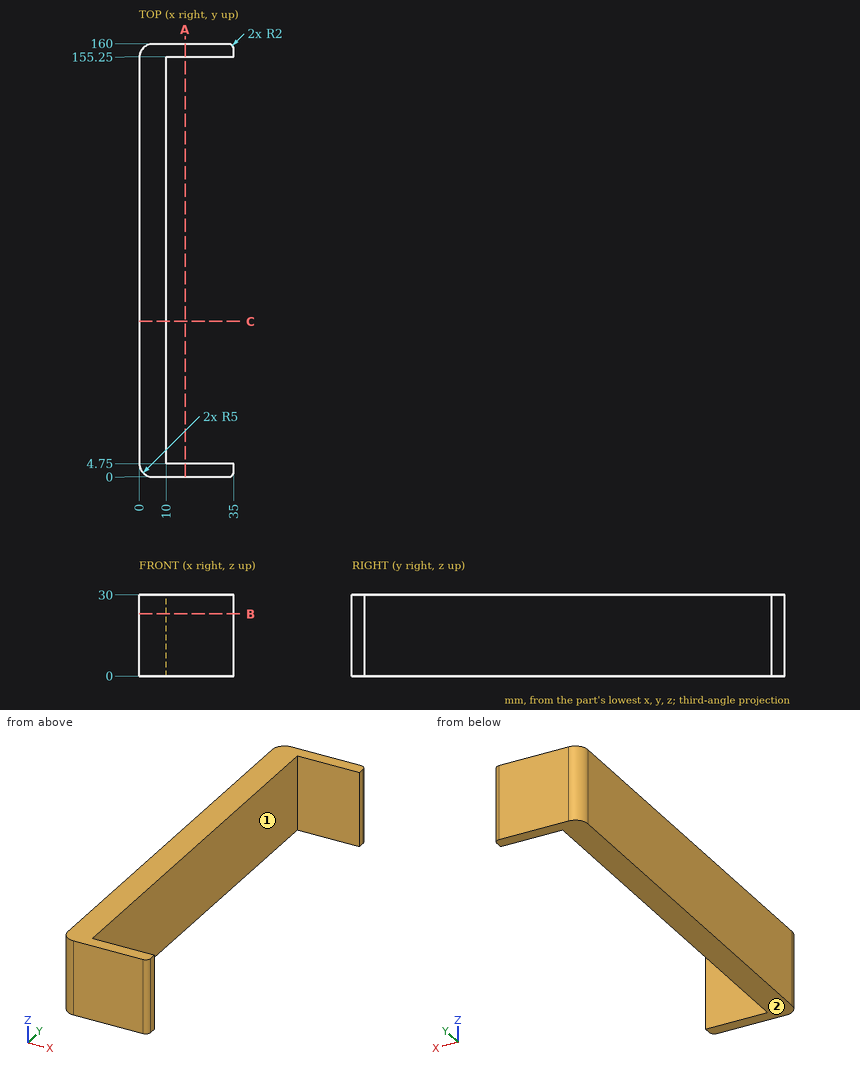
Verification items for this drawing (mm, ordinates from the low corner). A direction names the side the tool comes from. Give positions to 0.01 mm unless a question says otherwise; leave off trailing zeros. Write each loop counter-clockwise with the first axis right and the second up, starting at its lowest first coordinate (ties: lowest second). Pieces come first, ordered by that corner, then holes. Notation, with made-up numbers: (75, 27) -> (102, 27) arc R19 cw to (102, 50) -> close; hole circle Ø7 at (63, -18). An arc over 180 degrees is marked (long way). Use one line per item in the form item = value.
Item 1: Sectioned sample at B-B on z = 23. Enter the section's corners in (x, y), plus the area to 4 significant figures.
Results list:
outline = (0, 5) arc R5 ccw to (5, 0) -> (33, 0) arc R2 ccw to (35, 2) -> (35, 4.75) -> (10, 4.75) -> (10, 155.25) -> (35, 155.25) -> (35, 158) arc R2 ccw to (33, 160) -> (5, 160) arc R5 ccw to (0, 155) -> close
area = 1,825 mm2
Item 2: Sectioned sample at A-A on x = 17. Enter the section's corners in (y, z).
Results list:
outline = (0, 0) -> (4.75, 0) -> (4.75, 30) -> (0, 30) -> close; (155.25, 0) -> (160, 0) -> (160, 30) -> (155.25, 30) -> close
Item 3: Depth check by flat-ended pin: pin 1 Ø15 at (y, z) = (59, 18.5) entering from +X. Enter the tip coordinate at first touch or a pass-through.
Results list:
pin_1 = 10
Item 4: Scan lines: line 1 (Y direction, x = 21, z = 3); line 2 (X direction, y = 84, z = 26.5). Record each from-to range of solid material in increasing order.
Results list:
line_1 = 0 to 4.75, 155.25 to 160
line_2 = 0 to 10
Item 5: Access from +Z, -Z, +X, -X, +Y, -Y to the whole of each face (thin tool, end or side, straight path). Record for the marked faces 1 and 2.
Results list:
face_1 = +Z, -Z, +X
face_2 = -Z, +X, -X, +Y, -Y
Item 6: Sectioned sample at C-C on y = 57.5. Enter the section's corners in (x, z).
Results list:
outline = (0, 0) -> (10, 0) -> (10, 30) -> (0, 30) -> close
